Autodesk Inventor part; units mm, degrees
ref_plane "YZ Plane" through (0, 0, 0) normal (1, 0, 0) x (0, 1, 0)
ref_plane "XZ Plane" through (0, 0, 0) normal (0, 1, 0) x (-1, 0, 0)
ref_plane "XY Plane" through (0, 0, 0) normal (0, 0, 1) x (1, 0, 0)
sketch "スケッチ1" plane through (0, 0, 0) normal (0, 0, 1) x (1, 0, 0)
  circle A0 centre (0, 0) radius 23.5
  line L0 (0, 0) -> (0, 60)
  line L1 (0, 60) -> (25, 60)
  line L2 (25, 60) -> (25, 110)
  line L3 (25, 110) -> (0, 110)
  line L4 (0, 110) -> (0, 60)
  line L5 (25, 60) -> (23.4927, -0.5845)
  line L6 (0, 60) -> (-25, 60)
  line L7 (-25, 60) -> (-25, 110)
  line L8 (-25, 110) -> (0, 110)
  line L9 (-25, 60) -> (-23.4927, -0.5845)
  point P0 (-23.4927, -0.5845)
  dimension "d0" = 47
  dimension "d1" = 60
  dimension "d2" = 50
  dimension "d3" = 25
extrude "プレート1" add sketch "スケッチ1" along normal blind 2
sketch "スケッチ2" plane through (27, 60, -2) normal (1, 0, 0) x (0, 1, 0)
  line L0 (50, 0) -> (0, 0)
  line L1 (0, 0) -> (0, -34)
  line L2 (0, -34) -> (50, -34)
  line L3 (50, -34) -> (50, 0)
edge flange "フランジ1" height 38 angle 90 thickness 2 bend radius 2 thickness toward (1, 0, 0) relief tear relief width 2 relief depth 1 edges at (25, 85, 0) wall of the first edge with corners at (27, 110, -2) (27, 60, -2) (27, 60, -36) (27, 110, -36)
bend "曲げ1"
corner "コーナー1"
sketch "スケッチ3" plane through (-27, 110, -2) normal (-1, 0, 0) x (0, -1, 0)
  line L0 (50, 0) -> (0, 0)
  line L1 (0, 0) -> (0, -34)
  line L2 (0, -34) -> (50, -34)
  line L3 (50, -34) -> (50, 0)
edge flange "フランジ2" height 38 angle 90 thickness 2 bend radius 2 thickness toward (-1, 0, 0) relief tear relief width 2 relief depth 1 edges at (-25, 85, 0) wall of the first edge with corners at (-27, 60, -2) (-27, 110, -2) (-27, 110, -36) (-27, 60, -36)
bend "曲げ2"
corner "コーナー2"
sketch "スケッチ4" plane through (0, 0, 2) normal (0, 0, 1) x (1, 0, 0)
  circle A0 centre (0, 0) radius 10.1
  dimension "d25" = 20.2
extrude "押し出し1" [suppressed]
sketch "スケッチ5" plane through (0, 0, 2) normal (0, 0, 1) x (1, 0, 0)
  circle A0 centre (0, 0) radius 15.18
  point P0 (0, 15.18)
  point P1 (-13.1463, 7.59)
  point P2 (-13.1463, -7.59)
  point P3 (0, -15.18)
  point P4 (13.1463, -7.59)
  point P5 (13.1463, 7.59)
  dimension "d28" = 30.36
  dimension "d31" = 360
hole "穴1" [suppressed]
sketch "スケッチ6" plane through (29, 60, -36) normal (1, 0, 0) x (0, 0, -1)
  line L0 (0, 0) -> (0, 50)
  line L1 (0, 10) -> (-34, 10)
  line L2 (-34, 50) -> (-34, 0)
  line L3 (0, 0) -> (-34, 0)
  line L4 (0, 50) -> (-34, 50)
  line L5 (-10, 50) -> (-10, 10)
  point P0 (-36, -60)
  point P1 (-10, 20)
  point P2 (-10, 40)
  point P3 (-36, 50)
  dimension "d40" = 10
  dimension "d42" = 10
  dimension "d43" = 20
  dimension "d69" = 26
hole "穴2" at (29, 80, -26) at (29, 100, -26) direction (-1, 0, 0) diameter 3.2 end through all
sketch "スケッチ7" plane through (0, 0, 0) normal (0, 0, -1) x (-1, 0, 0)
  point P0 (0, 0)
  point P1 (0, 0)
hole "穴3" at (0, 0, 0) direction (0, 0, 1) diameter 3.1 end through all
sketch "スケッチ8" plane through (0, 0, 2) normal (0, 0, 1) x (1, 0, 0)
  line L0 (-15, 100) -> (15, 100)
  line L1 (15, 100) -> (15, 60)
  line L2 (15, 60) -> (-15, 60)
  line L3 (-15, 60) -> (-15, 100)
  line L4 (25, 110) -> (25, 60)
  line L5 (-25, 60) -> (-25, 110)
  line L6 (-25, 110) -> (25, 110)
  circle A0 centre (0, 0) radius 1.55
  circle A1 centre (0, 0) radius 13.5
  line L7 (-14.4993, 40) -> (-13.4958, -0.3358)
  line L8 (-23.4927, -0.5845) -> (-25, 60)
  line L9 (13.4958, -0.3358) -> (14.4993, 40)
  line L10 (25, 60) -> (23.4927, -0.5845)
  line L11 (14.4993, 40) -> (-14.4993, 40)
  dimension "d58" = 10
  dimension "d59" = 10
  dimension "d60" = 10
  dimension "d61" = 40
  dimension "d63" = 10
  dimension "d64" = 20
extrude "押し出し2" [suppressed]
fillet "フィレット1" [suppressed]
fillet "フィレット2" radius 2 4 edges at (28, 60, -36) (28, 110, -36) (-28, 110, -36) (-28, 60, -36)
equation "\"d38\" = Thickness"
equation "\"d56\" = Thickness"
equation "\"d4\" = Thickness"
equation "\"d5\" = BendReliefWidth"
equation "\"d6\" = BendReliefDepth"
equation "\"d7\" = MinimumRemnant"
equation "\"d8\" = TransitionRadius"
equation "\"d11\" = BendRadius"
equation "\"d12\" = CornerReliefSize"
equation "\"d13\" = GapSize"
equation "\"d14\" = JacobiRadiusSize"
equation "\"d15\" = BendReliefWidth"
equation "\"d16\" = BendReliefDepth"
equation "\"d17\" = MinimumRemnant"
equation "\"d18\" = TransitionRadius"
equation "\"d21\" = BendRadius"
equation "\"d22\" = CornerReliefSize"
equation "\"d23\" = GapSize"
equation "\"d24\" = JacobiRadiusSize"
equation "\"BendRadius\" = Thickness"
equation "\"BendReliefWidth\" = Thickness"
equation "\"BendReliefDepth\" = 0.5 * Thickness"
equation "\"CornerReliefSize\" = 4 * Thickness"
equation "\"MinimumRemnant\" = 2 * Thickness"
equation "\"TransitionRadius\" = BendRadius"
equation "\"JacobiRadiusSize\" = BendRadius"
equation "\"GapSize\" = Thickness"
properties part number "servoplate2_forR3" material "アルミニウム 6061"
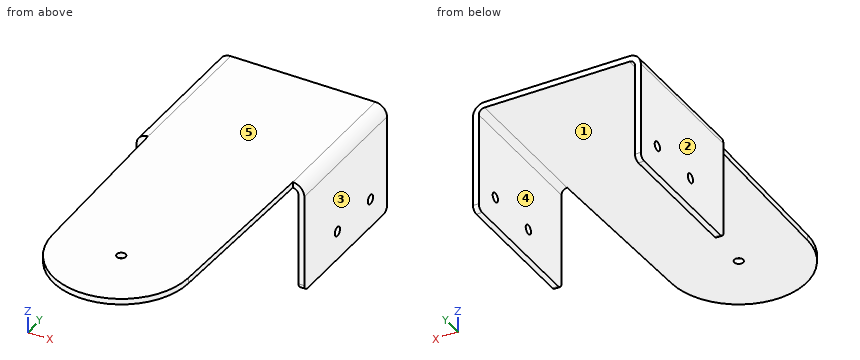
Geometry check sheet. Reference: the model listing, model coordinates, mm. Face numbers are marked on the shaded views. A direction names the side the tool comes from. Round coordinates to 2 decimals unless told otherwise and drop trailing zeros. Loops run counter-clockwise (first coordinate to the right, second up) from the corner with the lowest first, then second, coordinate; pieces in that order, holes last.
Item 1: Cross-section at B-B on y = 100. Record the boundary of the cut face in (x, z), then the cut area to 3 significant figures.
Item 2: Access from +Z, -Z, +X, -X, +Y, -Y to the whole of each face (thin tool, end or side, straight path). Record for the marked faces 1 and 2.
Item 3: Cross-section at C-C on x = 0. Record the boundary of the cut face in (y, z).
Item 4: Thickness scan on line 1 (Y direction, x = -28, z = -26); line 2 (X direction, y = 66.5, z = -18.5); line 3 (Y direction, x = 0, z = 1.15). Record the ranges inside material, lowest first.
Item 5: Gauge pin test, flat ends, axial feed: pin 1 (2 mm diameter, centred on x = 27, z = -13.5, fed in from -Y); pin 2 (3 mm diameter, centred on y = 80, z = -26, fed in from -X); pin 3 (4 mm diameter, centred on x = -18.5, y = 83, fed in from -Z). Record the tip position at first contact, or that the pin passes through.
Item 6: Cross-section at D-D on z = -26. Record the boundary of the cut face in (x, y).
Item 7: Mould release check, pull along X, two halves, no side actions. Record for the marked faces 3, 4 and 5: pulls with the +X half, pulls with the -X half, needs draft (parallel to the pull), parting line crosses it, or undercut.
Item 8: Cross-section at A-A on z = -17.5. Record the boundary of the cut face in (x, y).
Answer sheet:
1. outline: (-29, -36) - (-27, -36) - (-27, -27.6) - (-29, -27.6) - close; (-29, -24.4) - (-27, -24.4) - (-27, -2) arc R2 cw to (-25, 0) - (25, 0) arc R2 cw to (27, -2) - (27, -24.4) - (29, -24.4) - (29, -2) arc R4 ccw to (25, 2) - (-25, 2) arc R4 ccw to (-29, -2) - close; (27, -36) - (29, -36) - (29, -27.6) - (27, -27.6) - close
1. area: 242 mm2
2. face 1: -Z, +Y, -Y
2. face 2: +Z, -Z, -X, +Y, -Y
3. outline: (-23.5, 0) - (-1.55, 0) - (-1.55, 2) - (-23.5, 2) - close; (1.55, 0) - (110, 0) - (110, 2) - (1.55, 2) - close
4. line 1: y = 60 to 78.4, 81.6 to 98.4, 101.6 to 110
4. line 2: x = -29 to -27, 27 to 29
4. line 3: y = -23.5 to -1.55, 1.55 to 110
5. pin 1: stops at y = 60
5. pin 2: passes through
5. pin 3: stops at z = 0
6. outline: (-29, 60) - (-27, 60) - (-27, 78.4) - (-29, 78.4) - close; (-29, 81.6) - (-27, 81.6) - (-27, 98.4) - (-29, 98.4) - close; (-29, 101.6) - (-27, 101.6) - (-27, 110) - (-29, 110) - close; (27, 60) - (29, 60) - (29, 78.4) - (27, 78.4) - close; (27, 81.6) - (29, 81.6) - (29, 98.4) - (27, 98.4) - close; (27, 101.6) - (29, 101.6) - (29, 110) - (27, 110) - close
7. face 3: pulls with the +X half
7. face 4: undercut
7. face 5: needs draft
8. outline: (-29, 60) - (-27, 60) - (-27, 110) - (-29, 110) - close; (27, 60) - (29, 60) - (29, 110) - (27, 110) - close
